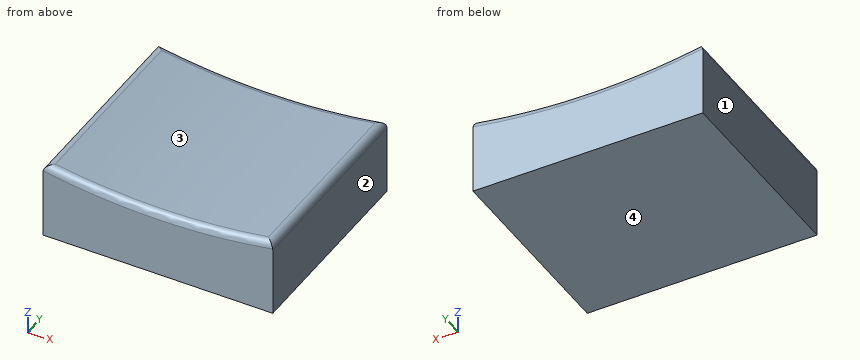
```python
from build123d import *

# Parameters (mm, degrees)
SKETCH1_W      = 8.3058
SKETCH1_H      = 7.3152
KEY_DEPTH      = 2.794
EXTRUDE2_DEPTH = 8.3152
FILLET1_R      = 0.254


with BuildPart() as part:
    # Sketch1 → key (new body)
    with BuildSketch(Plane.XY):
        Rectangle(SKETCH1_W, SKETCH1_H)
    extrude(amount=KEY_DEPTH)

    # Sketch2 → Extrude2 (cut, through all)
    with BuildSketch(Plane.XZ.offset(3.6576)):
        with BuildLine():
            ThreePointArc((-4.1529, 2.794), (0, 2.413613466), (4.1529, 2.794))
            Line((4.1529, 2.794), (-4.1529, 2.794))
        make_face()
    extrude(amount=-EXTRUDE2_DEPTH, mode=Mode.SUBTRACT)

    # Fillet1
    fillet1_edges = [part.edges().sort_by_distance(p)[0] for p in [
        (4.1529, 0, 2.794),
        (0, 3.6576, 2.413613466),
        (0, -3.6576, 2.413613466),
        (-4.1529, 0, 2.794),
    ]]
    fillet(fillet1_edges, radius=FILLET1_R)


solid = part.part
```
Work out the finished part from the listing and answer in its coordinate system (mm). Face numbers are marked on the shaded views. Coordinates: 2 decimals unless noted, no trailing zeros. Order: outer loops, then holes, each group sorted by start corner. A loop starts at its lowest first (then second) coordinate and runs counter-clockwise, first axis right, second up. Notation, with made-up numbers: (0.5, -14) - (45.5, -14) arc R17 ccw to (45.5, -9) - close; hole circle Ø4 at (82.25, 77). An arc over 180 degrees is marked (long way). Answer as a JSON object with one key per item and string values.
1. The mould has two halves that part along X. Classify the marked faces 1, 2, 3 and 4: +X half, -X half, draft (parallel to the pull), parting line (faces both ways), or undercut.
Output values:
{"face 1": "-X half", "face 2": "+X half", "face 3": "undercut", "face 4": "draft"}
2. This flat-tipped pin is pushed along its axis until it touches: P1, Ø3, axis at x = 0, y = -1.5, coming from the +Z side. Where does it stop, or does it pass through?
Output values:
{"P1": "stops at z = 2.46"}
3. Find section A-A on y = 2.25. Determine the outline of the cut face in (x, z), plus the area to 3 significant figures.
Output values:
{"outline": "(-4.15, 0) - (4.15, 0) - (4.15, 2.49) arc R0.25 ccw to (3.86, 2.74) arc R22.86 cw to (-3.86, 2.74) arc R0.25 ccw to (-4.15, 2.49) - close", "area": "21.1 mm²"}
4. Consider line 1 (Z direction, x = -0.5, y = -3.5); line 2 (Z direction, x = 1.5, y = -0.5); line 3 (Y direction, x = -1, z = 2.35). Determine where each line is inside the solid, lowest interval first.
Output values:
{"line 1": "z = 0 to 2.4", "line 2": "z = 0 to 2.46", "line 3": "y = -3.59 to 3.59"}
5. Find section B-B on x = 0. Determine the outline of the cut face in (y, z), plus the area to 3 significant figures.
Output values:
{"outline": "(-3.66, 0) - (3.66, 0) - (3.66, 2.16) arc R0.25 ccw to (3.4, 2.41) - (-3.4, 2.41) arc R0.25 ccw to (-3.66, 2.16) - close", "area": "17.6 mm²"}
